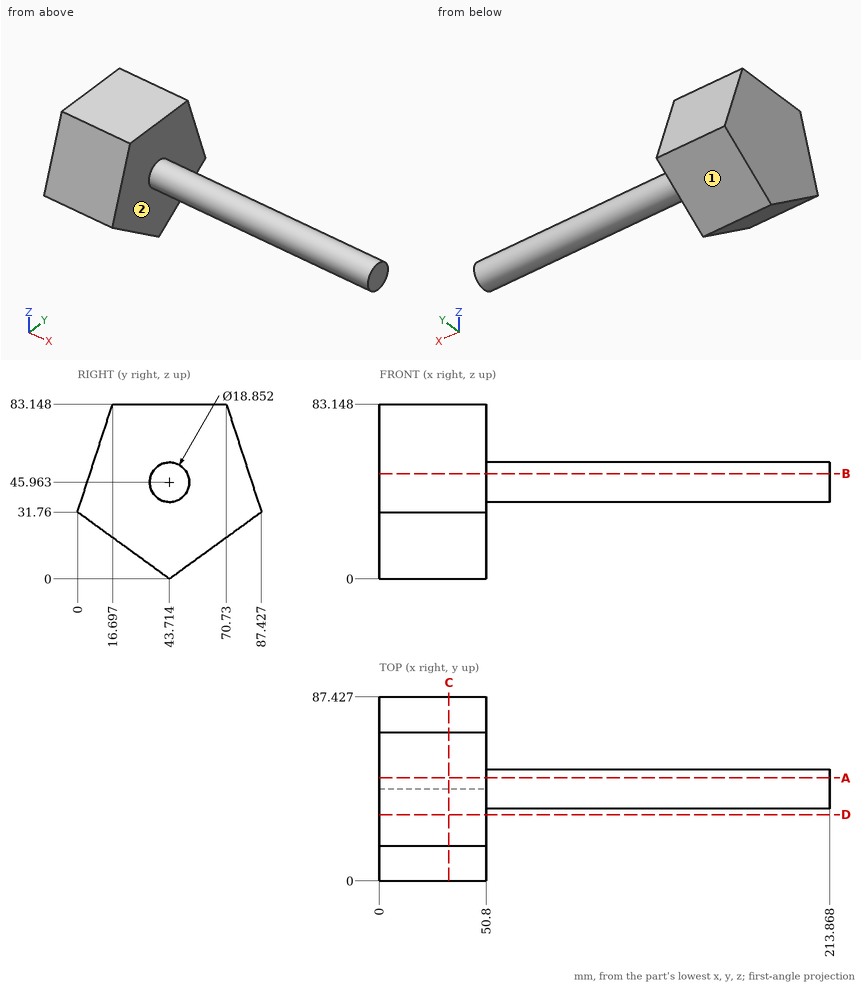
Could you check a few things on this drawing? It's one solid part, dimensions in mm from its lowest x, y, z. A direction names the side the tool comes from. Give positions to 0.01 mm unless a question says otherwise; leave off trailing zeros. Order: outer loops, then holes, each group sorted by start corner. A loop starts at its lowest first (then second) coordinate and runs counter-clockwise, first axis right, second up. Notation, with made-up numbers: M 15.5,59 L 63.5,59 A15 ccw 63.5,71 Z; hole C 27,32.25 d9. An arc over 180 degrees is marked long. Use one line per item in the form item = value. Start each with the question number.
Item 1: If we section it at D-D (y = 31.5): Write out the boundary of the cut face in (x, z).
Item 2: If I drill on line 1 along X through (y, z) = (52.5, 37); line 2 along Z through (x, y) = (117.5, 36.5) (1 decimal); line 3 along Y through (x, z) = (135.5, 44) (1 decimal), over which ranges is the centre line in solid material (lowest first)?
Item 3: If we section it at A-A (y = 49): Write out the boundary of the cut face in (x, z), then the cut area to 3 significant figures.
Item 4: If we section it at B-B (z = 50): Write out the boundary of the cut face in (x, y) (1 decimal), then the cut area to 3 significant figures.
Item 5: Will these pins go through, and if not, where does the flat tip stop? pin 1 Ø10 at (x, z) = (54, 12) entering from -Y; pin 2 Ø4 at (x, y) = (40.5, 64.5) entering from -Z; pin 3 Ø10 at (x, y) = (83, 47) entering from +Z.
Item 6: For the marked faces 1 and 2, which set-ups out of +Z, -Z, +X, -X, +Y, -Y let a thin tool reach every point of the face, with its end or its side?
Item 7: If we section it at C-C (x = 33): Write out the boundary of the cut face in (y, z).
Outcome:
q1.outline = M 0,8.87 L 50.8,8.87 L 50.8,83.15 L 0,83.15 Z
q2.line_1 = 0 to 50.8
q2.line_2 = 39.9 to 52
q2.line_3 = 34.5 to 52.9
q3.outline = M 0,3.84 L 50.8,3.84 L 50.8,38.16 L 213.87,38.16 L 213.87,53.77 L 50.8,53.77 L 50.8,83.15 L 0,83.15 Z
q3.area = 6,570 mm2
q4.outline = M 0,5.9 L 50.8,5.9 L 50.8,35.2 L 213.9,35.2 L 213.9,52.2 L 50.8,52.2 L 50.8,81.5 L 0,81.5 Z
q4.area = 6,620 mm2
q5.pin_1 = 21.91
q5.pin_2 = 13.65
q5.pin_3 = 55.39
q6.face_1 = -Z, +X, -X, +Y
q6.face_2 = +X
q7.outline = M 0,31.76 L 43.71,0 L 87.43,31.76 L 70.73,83.15 L 16.7,83.15 Z
